Work out the finished part from the listing and answer in its coordinate system (mm). Give positions to 0.01 mm unless a question says otherwise; leave off trailing zeros. Write each loop counter-clockwise with the first axis right and the second up, starting at its lowest first coordinate (ties: lowest second). Pieces come first, ordered by that corner, then holes. Notation, with made-up numbers: (56.25, 24.25) -> (76.25, 24.25) arc R29 cw to (76.25, 59.25) -> close; hole circle Ø5 at (43.25, -11.75). An arc over 180 degrees is marked (long way). Use a Markdown table: item, result. Add a question column.
Q1. Consider line 1 (X direction, y = 100, z = 1.15); line 2 (Y direction, x = 10, z = 1.5); line 3 (X direction, y = 101, z = 1.6). Determine where each line is inside the solid, lowest interval first.
Q2. Section A-A, the plane x = 10 is taken. Give the vertices of the cut face in (y, z).
Q3. For a pull along X with two mould halves and no side action, classify faces 1 (the face through (74, 61, 0)), 2 (the face through (138, 20, 1)) as pulls with the +X half, pulls with the -X half, needs draft (parallel to the pull), parting line crosses it, or undercut.
Q4. Section B-B, the plane y = 100 is taken. Give the vertices of the cut face in (x, z), plus the area to 3 significant figures.
from build123d import *

# Parameters (mm, degrees)
SKETCH001_W     = 139
SKETCH001_H     = 99
PAD_DEPTH       = 2
SKETCH003_R     = 2
POCKET_DEPTH    = 5
SKETCH004_R     = 2
POCKET001_DEPTH = 5
SKETCH005_R     = 2
POCKET002_DEPTH = 5
SKETCH006_R     = 2
POCKET003_DEPTH = 5


with BuildPart() as part:
    # Sketch001 → Pad (new body)
    with BuildSketch(Plane.XY):
        with Locations((75, 60)):
            Rectangle(SKETCH001_W, SKETCH001_H)
    extrude(amount=PAD_DEPTH)

    # Sketch003 → Pocket (cut)
    with BuildSketch(Plane.XY):
        with Locations((10, 20)):
            Circle(SKETCH003_R)
    extrude(amount=POCKET_DEPTH, mode=Mode.SUBTRACT)

    # Sketch004 → Pocket001 (cut)
    with BuildSketch(Plane.XY):
        with Locations((10, 100)):
            Circle(SKETCH004_R)
    extrude(amount=POCKET001_DEPTH, mode=Mode.SUBTRACT)

    # Sketch005 → Pocket002 (cut)
    with BuildSketch(Plane.XY):
        with Locations((140, 20)):
            Circle(SKETCH005_R)
    extrude(amount=POCKET002_DEPTH, mode=Mode.SUBTRACT)

    # Sketch006 → Pocket003 (cut)
    with BuildSketch(Plane.XY):
        with Locations((140, 100)):
            Circle(SKETCH006_R)
    extrude(amount=POCKET003_DEPTH, mode=Mode.SUBTRACT)


solid = part.part
Result set:
| question | item | result |
|---|---|---|
| 1 | line 1 | x = 5.5 to 8, 12 to 138, 142 to 144.5 |
| 1 | line 2 | y = 10.5 to 18, 22 to 98, 102 to 109.5 |
| 1 | line 3 | x = 5.5 to 8.27, 11.73 to 138.27, 141.73 to 144.5 |
| 2 | outline | (10.5, 0) -> (18, 0) -> (18, 2) -> (10.5, 2) -> close; (22, 0) -> (98, 0) -> (98, 2) -> (22, 2) -> close; (102, 0) -> (109.5, 0) -> (109.5, 2) -> (102, 2) -> close |
| 3 | face 1 | needs draft |
| 3 | face 2 | undercut |
| 4 | outline | (5.5, 0) -> (8, 0) -> (8, 2) -> (5.5, 2) -> close; (12, 0) -> (138, 0) -> (138, 2) -> (12, 2) -> close; (142, 0) -> (144.5, 0) -> (144.5, 2) -> (142, 2) -> close |
| 4 | area | 262 mm2 |
